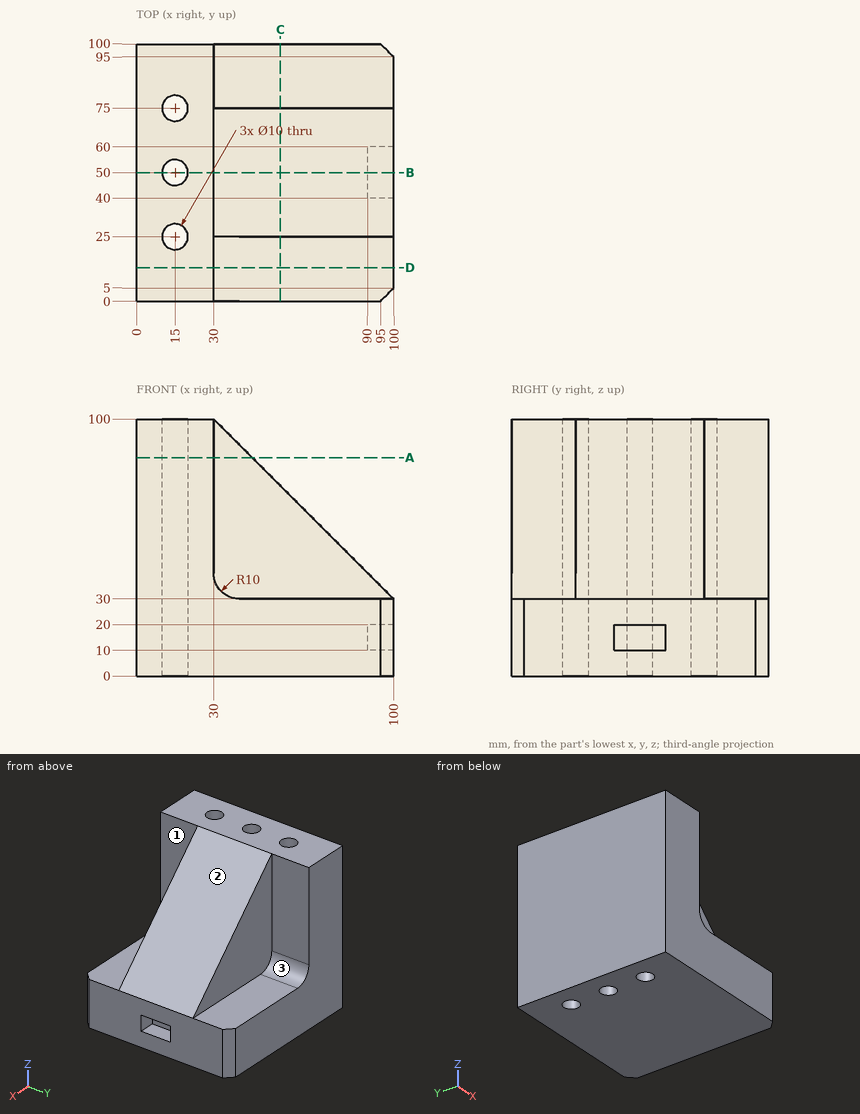
For this review, use the dimensioned drawing (mm, ordinates from the lowest corner) and the shaded views. A direction names the side the tool comes from. Round coordinates to 2 decimals unless told otherwise and drop trailing zeros. Order: outer loops, then holes, each group sorted by start corner. A loop starts at its lowest first (then second) coordinate and runs counter-clockwise, first axis right, second up. Notation, with made-up numbers: (30.5, -15) -> (67.5, -15) arc R33 cw to (67.5, 15) -> close; hole circle Ø5 at (75, 33). An arc over 180 degrees is marked (long way). Put each result on its own line as item: value.
Q1. Add section B-B on y = 50. Write out the cut boundary in (x, z), plus the area to 3 significant figures.
Check result:
outline: (0, 0) -> (10, 0) -> (10, 100) -> (0, 100) -> close; (20, 0) -> (100, 0) -> (100, 10) -> (90, 10) -> (90, 20) -> (100, 20) -> (100, 30) -> (30, 100) -> (20, 100) -> close
area: 6,450 mm2
Q2. Machinability: for the marked faces 1, 2 and 3, which of the approach directions +Z, -Z, +X, -X, +Y, -Y give a long, thin tool a straight path to every point of the face, cutting with its end or side? Answer none if there is none.
Check result:
face 1: +Z, +X, -Y
face 2: +Z, +X, +Y, -Y
face 3: +Z, +X, +Y
Q3. Insertion check: pin 1 Ø4 at (x, y) = (61, 11.5) entering from +Z; pin 2 Ø7.5 at (y, z) = (7, 59) entering from +X; pin 3 Ø1.5 at (x, z) = (38.5, 41.5) entering from -Y; pin 4 Ø8 at (x, y) = (15, 75) entering from -Z. Each pin has a flat end and moves straight along its axis. Give the tip position at first contact, or say it passes through.
Check result:
pin 1: z = 30
pin 2: x = 30
pin 3: y = 25
pin 4: through
Q4. Add section C-C on x = 56. Write out the cut boundary in (y, z).
Check result:
outline: (0, 0) -> (100, 0) -> (100, 30) -> (75, 30) -> (75, 74) -> (25, 74) -> (25, 30) -> (0, 30) -> close
Q5. Add section D-D on y = 13. Write out the cut boundary in (x, z).
Check result:
outline: (0, 0) -> (100, 0) -> (100, 30) -> (40, 30) arc R10 cw to (30, 40) -> (30, 100) -> (0, 100) -> close
Q6. Add section A-A on z = 85. Write out the cut boundary in (x, y), plus the area to 3 significant figures.
Check result:
outline: (0, 0) -> (30, 0) -> (30, 25) -> (45, 25) -> (45, 75) -> (30, 75) -> (30, 100) -> (0, 100) -> close; hole circle Ø10 at (15, 25); hole circle Ø10 at (15, 50); hole circle Ø10 at (15, 75)
area: 3,510 mm2
Q7. For probe 1 along Y at (x, z) = (15, 40); probe 2 along Y at (x, z) = (18.5, 80); probe 3 along Y at (x, z) = (61, 48), list the stretches that pass through material, from the lowest coordinate up. Write a range as [from, to].
Check result:
probe 1: [0, 20], [30, 45], [55, 70], [80, 100]
probe 2: [0, 21.43], [28.57, 46.43], [53.57, 71.43], [78.57, 100]
probe 3: [25, 75]
